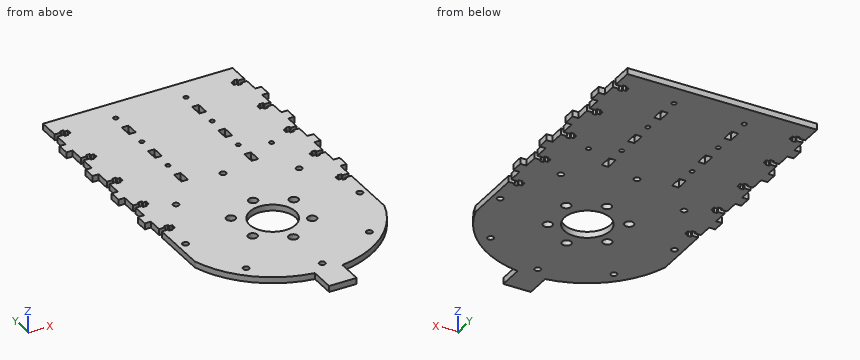
```python
from build123d import *

# Parameters (mm, degrees)
SKETCH_1_R          = 2.28339151
EXTRUDE_1_DEPTH     = 4
SKETCH_3_R          = 3
SKETCH_3_R_2        = 15
SKETCH_3_R_3        = 2
CUT_EXTRUDE_1_DEPTH = 4
SKETCH_6_R          = 1.5
SKETCH_6_W          = 4.4
SKETCH_6_H          = 8.4
CUT_EXTRUDE_3_DEPTH = 4
SKETCH_7_R          = 1.5
CUT_EXTRUDE_5_DEPTH = 10
EXTRUDE_2_DEPTH     = 4


with BuildPart() as part:
    # 草图1 → 凸台-拉伸1 (new body)
    with BuildSketch(Plane.XY):
        Polygon((145, 46.5), (149, 46.5), (149, 45.15), (151.6, 45.15), (151.6, 46.5), (153.6, 46.5), (153.6, 49.5), (151.6, 49.5), (151.6, 50.85), (149, 50.85), (149, 49.5), (145, 49.5), (145, 59), (141, 59), (141, 67), (145, 67), (145, 76.5), (149, 76.5), (149, 75.15), (151.6, 75.15), (151.6, 76.5), (153.6, 76.5), (153.6, 79.5), (151.6, 79.5), (151.6, 80.85), (149, 80.85), (149, 79.5), (145, 79.5), (145, 89), (141, 89), (141, 97), (145, 97), (145, 106.5), (149, 106.5), (149, 105.15), (151.6, 105.15), (151.6, 106.5), (153.6, 106.5), (153.6, 109.5), (151.6, 109.5), (151.6, 110.85), (149, 110.85), (149, 109.5), (145, 109.5), (145, 123), (269, 123), (269, 109.5), (265, 109.5), (265, 110.85), (262.4, 110.85), (262.4, 109.5), (260.4, 109.5), (260.4, 106.5), (262.4, 106.5), (262.4, 105.15), (265, 105.15), (265, 106.5), (269, 106.5), (269, 97), (273, 97), (273, 89), (269, 89), (269, 79.5), (265, 79.5), (265, 80.85), (262.4, 80.85), (262.4, 79.5), (260.4, 79.5), (260.4, 76.5), (262.4, 76.5), (262.4, 75.15), (265, 75.15), (265, 76.5), (269, 76.5), (269, 67), (273, 67), (273, 59), (269, 59), (269, 49.5), (265, 49.5), (265, 50.85), (262.4, 50.85), (262.4, 49.5), (260.4, 49.5), (260.4, 46.5), (262.4, 46.5), (262.4, 45.15), (265, 45.15), (265, 46.5), (269, 46.5), (269, 37), (273, 37), (273, 29), (269, 29), (269, 19.5), (265, 19.5), (265, 20.85), (262.4, 20.85), (262.4, 19.5), (260.4, 19.5), (260.4, 16.5), (262.4, 16.5), (262.4, 15.15), (265, 15.15), (265, 16.5), (269, 16.5), (269, 7), (273, 7), (273, -1), (269, -1), (269, -10.5), (265, -10.5), (265, -9.15), (262.4, -9.15), (262.4, -10.5), (260.4, -10.5), (260.4, -13.5), (262.4, -13.5), (262.4, -14.85), (265, -14.85), (265, -13.5), (269, -13.5), (269, -27), (269, -97), (145, -97), (145, -27), (145, -13.5), (149, -13.5), (149, -14.85), (151.6, -14.85), (151.6, -13.5), (153.6, -13.5), (153.6, -10.5), (151.6, -10.5), (151.6, -9.15), (149, -9.15), (149, -10.5), (145, -10.5), (145, -1), (141, -1), (141, 7), (145, 7), (145, 16.5), (149, 16.5), (149, 15.15), (151.6, 15.15), (151.6, 16.5), (153.6, 16.5), (153.6, 19.5), (151.6, 19.5), (151.6, 20.85), (149, 20.85), (149, 19.5), (145, 19.5), (145, 29), (141, 29), (141, 37), (145, 37), align=None)
        with Locations((262.4, -88.911124512)):
            Circle(SKETCH_1_R, mode=Mode.SUBTRACT)
    extrude(amount=EXTRUDE_1_DEPTH)

    # 草图3 → 切除-拉伸1 (cut)
    with BuildSketch(Plane.XY.offset(4)):
        with Locations((207, -55.75)):
            Circle(SKETCH_3_R)
        with Locations((226.485571585, -43.25)):
            Circle(SKETCH_3_R)
        with Locations((207, -32)):
            Circle(SKETCH_3_R_2)
        with Locations((264, -32)):
            Circle(SKETCH_3_R_3)
        with Locations((186.43189666, -20.125)):
            Circle(SKETCH_3_R)
        with Locations((227.56810334, -20.125)):
            Circle(SKETCH_3_R)
        with Locations((187.514428415, -43.25)):
            Circle(SKETCH_3_R)
        with Locations((207, -9.5)):
            Circle(SKETCH_3_R)
        with Locations((247.305086528, -72.305086528)):
            Circle(SKETCH_3_R_3)
        with Locations((207, -89)):
            Circle(SKETCH_3_R_3)
        with Locations((166.694913472, -72.305086528)):
            Circle(SKETCH_3_R_3)
        with Locations((150, -32)):
            Circle(SKETCH_3_R_3)
        with Locations((166.694913472, 8.305086528)):
            Circle(SKETCH_3_R_3)
        with Locations((207, 25)):
            Circle(SKETCH_3_R_3)
        with Locations((247.305086528, 8.305086528)):
            Circle(SKETCH_3_R_3)
    extrude(amount=-CUT_EXTRUDE_1_DEPTH, mode=Mode.SUBTRACT)

    # 草图6 → 切除-拉伸3 (cut)
    with BuildSketch(Plane.XY.offset(4)):
        with Locations((184, 108)):
            Circle(SKETCH_6_R)
        with Locations((184, 78)):
            Circle(SKETCH_6_R)
        with Locations((184, 48)):
            Circle(SKETCH_6_R)
        with Locations(Location((230, 48, 0), (0, 0, 180))):
            Circle(SKETCH_6_R)
        with Locations(Location((230, 78, 0), (0, 0, 180))):
            Circle(SKETCH_6_R)
        with Locations(Location((230, 108, 0), (0, 0, 180))):
            Circle(SKETCH_6_R)
        with Locations((184, 93)):
            Rectangle(SKETCH_6_W, SKETCH_6_H)
        with Locations((184, 63)):
            Rectangle(SKETCH_6_W, SKETCH_6_H)
        with Locations((184, 33)):
            Rectangle(SKETCH_6_W, SKETCH_6_H)
        with Locations((230, 33)):
            Rectangle(SKETCH_6_W, SKETCH_6_H)
        with Locations((230, 63)):
            Rectangle(SKETCH_6_W, SKETCH_6_H)
        with Locations((230, 93)):
            Rectangle(SKETCH_6_W, SKETCH_6_H)
    extrude(amount=-CUT_EXTRUDE_3_DEPTH, mode=Mode.SUBTRACT)

    # 草图7 → 切除-拉伸5 (cut)
    with BuildSketch(Plane.XY.offset(4)):
        with Locations((247.644363383, 40.735296654)):
            Circle(SKETCH_7_R)
        with BuildLine():
            Line((142, -32), (85.31125556, -32))
            ThreePointArc((85.31125556, -32), (207, -153.68874444), (328.68874444, -32))
            Line((328.68874444, -32), (272, -32))
            ThreePointArc((272, -32), (207, -97), (142, -32))
        make_face()
    extrude(amount=-CUT_EXTRUDE_5_DEPTH, mode=Mode.SUBTRACT)

    # 草图8 → 凸台-拉伸2 (add)
    with BuildSketch(Plane.XY.offset(4)):
        Polygon((198, -112.71554622), (207, -112.71554622), (216, -112.71554622), (216, -91), (198, -91), align=None)
    extrude(amount=-EXTRUDE_2_DEPTH)


solid = part.part
```
Check sheet for the modelled part. Datum: model origin and axes. Units: mm. Round coordinates to 2 decimals unless told otherwise and drop trailing zeros. Write each loop counter-clockwise with the first axis right and the second up, starting at its lowest first coordinate (ties: lowest second). Pieces come first, ordered by that corner, then holes. Notation, with made-up numbers: M 33,-28 L 88,-28 A18 ccw 88,-6 Z; hole C 22,36 d7. An arc over 180 degrees is marked long. Write item = value, one per line. Start each with the question number.
1. Section check B-B, the plane y = -43.25. Record the cut outline in (x, z).
2. Gauge pin test, flat ends, axial feed: pin 1 (0.7 mm diameter, centred on y = 15.5, z = 2.5, fed in from -X); pin 2 (1.6 mm diameter, centred on x = 153, z = 2, fed in from -Y); pin 3 (2 mm diameter, centred on x = 261.5, z = 1.5, fed in from -Y); pin 4 (3 mm diameter, centred on x = 207, y = -89, fed in from +Z). Record the tip position at first contact, or that the pin passes through.
3. Section check D-D, the plane y = 100. Record the cut outline in (x, z), then the cut area to 3 significant figures.
4. Scan lines: line 1 (Y direction, x = 207, z = 3.1); line 2 (X direction, y = 94, z = 0.4); line 3 (X direction, y = -100.5, z = 2.05). Record each from-to range of solid material in increasing order. Write a range as [from, to].
5. Section check C-C, the plane z = 1.35. State how many separate pieces and enclosed holes the cut face has, then the cut area to 3 significant figures.
6. Section check A-A, the plane y = 32.5. Record the cut outline in (x, z).
Results found:
q1.outline = M 145,0 L 184.51,0 L 184.51,4 L 145,4 Z; M 190.51,0 L 197.08,0 L 197.08,4 L 190.51,4 Z; M 216.92,0 L 223.49,0 L 223.49,4 L 216.92,4 Z; M 229.49,0 L 269,0 L 269,4 L 229.49,4 Z
q2.pin_1 = 145
q2.pin_2 = -69.35
q2.pin_3 = -68.92
q2.pin_4 = through
q3.outline = M 145,0 L 269,0 L 269,4 L 145,4 Z
q3.area = 496 mm^2
q4.line_1 = [-112.72, -91], [-87, -58.75], [-52.75, -47], [-17, -12.5], [-6.5, 23], [27, 123]
q4.line_2 = [141, 181.8], [186.2, 227.8], [232.2, 273]
q4.line_3 = [198, 216]
q5.separate_pieces = 1
q5.enclosed_holes = 28
q5.area = 24,700 mm^2
q6.outline = M 141,0 L 181.8,0 L 181.8,4 L 141,4 Z; M 186.2,0 L 227.8,0 L 227.8,4 L 186.2,4 Z; M 232.2,0 L 273,0 L 273,4 L 232.2,4 Z
